Geometry: final body of the model. Coordinates: model frame, mm. Round coordinates to 2 decimals unless told otherwise and drop trailing zeros. Loops run counter-clockwise (first coordinate to the right, second up) from the corner with the lowest first, then second, coordinate; pieces in that order, holes last. Notation, with made-up numbers: M 42,2 L 69,2 A22 ccw 69,8 Z; hole C 6.5,-31.5 d5. An arc over 180 degrees is marked long. Answer as a JSON object with one key per item and string values.
```python
from build123d import *

# Parameters (mm, degrees)
SKETCH1_R           = 1.5
BOSS_EXTRUDE1_DEPTH = 2
SKETCH2_OUTSIDE_W   = 16.288
SKETCH2_OUTSIDE_H   = 15.71
SKETCH2_OUTSIDE_R   = 2.5
CUT_EXTRUDE1_DEPTH  = 2
CUT_EXTRUDE1_TAPER  = 60
SKETCH3_OUTSIDE_W   = 16.288
SKETCH3_OUTSIDE_H   = 15.71
SKETCH3_OUTSIDE_R   = 2.5
CUT_EXTRUDE2_DEPTH  = 2
CUT_EXTRUDE2_TAPER  = 60
FILLET1_R           = 0.05


with BuildPart() as part:
    # Sketch1 → Boss-Extrude1 (new body)
    with BuildSketch(Plane(origin=(0, 0, 0), x_dir=(1, 0, 0), z_dir=(0, 1, 0))):
        Polygon((-2.880337842, 0.192320694), (-1.606723528, -2.398285395), (1.273614314, -2.59060609), (2.880337842, -0.192320694), (1.606723528, 2.398285395), (-1.273614314, 2.59060609), align=None)
        Circle(SKETCH1_R, mode=Mode.SUBTRACT)
    extrude(amount=BOSS_EXTRUDE1_DEPTH)

    # Sketch2 outside → Cut-Extrude1 (cut)
    with BuildSketch(Plane(origin=(0, 2, 0), x_dir=(1, 0, 0), z_dir=(0, 1, 0))):
        Rectangle(SKETCH2_OUTSIDE_W, SKETCH2_OUTSIDE_H)
        Circle(SKETCH2_OUTSIDE_R, mode=Mode.SUBTRACT)
    extrude(amount=-CUT_EXTRUDE1_DEPTH, taper=CUT_EXTRUDE1_TAPER, mode=Mode.SUBTRACT)

    # Sketch3 outside → Cut-Extrude2 (cut)
    with BuildSketch(Plane.XZ):
        Rectangle(SKETCH3_OUTSIDE_W, SKETCH3_OUTSIDE_H)
        Circle(SKETCH3_OUTSIDE_R, mode=Mode.SUBTRACT)
    extrude(amount=-CUT_EXTRUDE2_DEPTH, taper=CUT_EXTRUDE2_TAPER, mode=Mode.SUBTRACT)

    # Fillet1
    fillet1_edges = [part.edges().sort_by_distance(p)[0] for p in [
        (-1.5, 0, 0),
        (-1.5, 2, 0),
    ]]
    fillet(fillet1_edges, radius=FILLET1_R)


solid = part.part
```
1) Line query: probe 1 along X at (y, z) = (0.8, 0.5); probe 2 along Z at (x, y) = (0, 1.4); probe 3 along X at (y, z) = (1.2, -0.5). Output: solid intervals per line, ascending.
Geometry results:
{"probe 1": "-2.54 to -1.41, 1.41 to 2.67", "probe 2": "-2.51 to -1.5, 1.5 to 2.51", "probe 3": "-2.67 to -1.41, 1.41 to 2.54"}
2) Cut plane A-A on y = 1.2. Return the cut outline in (x, z), and give its area (3 significant figures).
Geometry results:
{"outline": "M -2.88,-0.19 L -1.27,-2.59 L 1.61,-2.4 L 2.88,0.19 L 1.27,2.59 L -1.61,2.4 Z; hole C 0,0 d3", "area": "14.6 mm2"}
3) Cut plane C-C on z = 0. Return the cut outline in (x, y) (3 decimals).
Geometry results:
{"outline": "M -2.786,0.165 L -2.5,0 L -1.55,0 A0.05 ccw -1.5,0.05 L -1.5,1.95 A0.05 ccw -1.55,2 L -2.5,2 L -2.786,1.835 Z; M 1.5,0.05 A0.05 ccw 1.55,0 L 2.5,0 L 2.786,0.165 L 2.786,1.835 L 2.5,2 L 1.55,2 A0.05 ccw 1.5,1.95 Z"}
4) Pull-direction query (X, two-part tool) for faces 1 (the face through (0, 2, 2)), 2 (the face through (-1.5, 0.99, -0.07)), 3 (the face through (-2.63, 1.92, -0.17)); classes: +X half, -X half, draft (parallel to the pull), parting line (faces both ways), or undercut.
Geometry results:
{"face 1": "draft", "face 2": "undercut", "face 3": "-X half"}
5) First-contact query: pin 1 (2 mm diameter, centred on x = -0.5, z = 1.5, fed in from -Y). Flat tip, straight axial feed; report the tip coordinate or a pass-through.
Geometry results:
{"pin 1": "y = 0"}
